```python
from build123d import *

# Parameters (mm, degrees)
SKETCH1_R           = 16.0625
SKETCH1_R_2         = 18.5625
SKETCH1_R_3         = 1.6
SKETCH1_R_4         = 2.35
SKETCH1_R_5         = 2.5625
SKETCH1_R_6         = 7.5625
BOSS_EXTRUDE1_DEPTH = 5
FILLET1_R           = 15
FILLET2_R           = 30


with BuildPart() as part:
    # Sketch1 → Boss-Extrude1 (new body)
    with BuildSketch(Plane.XY):
        Polygon((-20, -31.5), (20, -31.5), (60, -13.814957213), (60, 13.141793742), (20, 31.5), (-20, 8.126584262), align=None)
        Circle(SKETCH1_R, mode=Mode.SUBTRACT)
        with Locations((40, 0)):
            Circle(SKETCH1_R_2, mode=Mode.SUBTRACT)
        with Locations((20, 11.209005776)):
            Circle(SKETCH1_R_3, mode=Mode.SUBTRACT)
        with Locations((20, -9.557095977)):
            Circle(SKETCH1_R_4, mode=Mode.SUBTRACT)
        with Locations((20, 21.918567686)):
            Circle(SKETCH1_R_5, mode=Mode.SUBTRACT)
        with Locations((20, -21.316811866)):
            Circle(SKETCH1_R_6, mode=Mode.SUBTRACT)
        with Locations((0.737105173, -21.316811866)):
            Circle(SKETCH1_R_3, mode=Mode.SUBTRACT)
        with Locations((-4.862894827, -21.316811866)):
            Circle(SKETCH1_R_3, mode=Mode.SUBTRACT)
    extrude(amount=BOSS_EXTRUDE1_DEPTH)

    # Fillet1
    fillet1_edges = [part.edges().sort_by_distance(p)[0] for p in [
        (20, -31.5, 2.5),
        (-20, 8.126584262, 2.5),
        (20, 31.5, 2.5),
        (60, 13.141793742, 2.5),
        (60, -13.814957213, 2.5),
    ]]
    fillet(fillet1_edges, radius=FILLET1_R)

    # Fillet2
    fillet2_edges = [part.edges().sort_by_distance(p)[0] for p in [
        (-20, -31.5, 2.5),
    ]]
    fillet(fillet2_edges, radius=FILLET2_R)


solid = part.part
```
Check sheet for the modelled part. Datum: model origin and axes. Units: mm. Give positions to 0.01 mm unless a question says otherwise; leave off trailing zeros. Order: outer loops, then holes, each group sorted by start corner. A loop starts at its lowest first (then second) coordinate and runs counter-clockwise, first axis right, second up. Notation, with made-up numbers: M 56,44 L 72,44 A22 cw 72,62 Z; hole C 29,-17.75 d3. An arc over 180 degrees is marked long. Answer in a Markdown table with one row per item. Add a question column.
Q1. Sectioned sample at C-C, the plane x = 20. Record the boundary of the cut face in (y, z), and give its area (3 significant figures).
Q2. Sectioned sample at A-A, the plane x = 34.5. Record the boundary of the cut face in (y, z), and give its area (3 significant figures).
Q3. Sectioned sample at B-B, the plane z = 2.9. Count the separate pieces of the cut face and the enclosed holes in it, and give its area (3 significant figures).
Q4. Thickness scan on L1, parallel to Y at x = 20, z = 3; L2, parallel to X at y = 8, z = 2.25; L3, parallel to Y at x = 0, z = 2.4. Record the ranges inside material, lowest first.
Q5. Gauge pin test, flat ends, axial feed: pin 1 Ø19.5 at (x, y) = (0, 0) entering from -Z; pin 2 Ø1 at (y, z) = (-18.5, 2.5) entering from +X; pin 3 Ø1.5 at (x, z) = (-11.5, 4) entering from +Y; pin 4 Ø1.5 at (x, z) = (19.5, 1.5) entering from -Y. Record the tip position at first contact, or that the pin passes through.
Q6. Release check for a two-part mould opening along Y. For faces 1 (the cylindrical face through (-10.979, -22.945, 2.535)), 2 (the cylindrical face through (19.653, 9.647, 2.465)), 3 (the flat face through (0.529, 20.123, 2.465)) record: released by +Y, released by -Y, zero draft, split by the parting line, or undercut.
Q7. Sectioned sample at D-D, the plane x = 0. Record the boundary of the cut face in (y, z), and give its area (3 significant figures).
Verdict:
| question | item | result |
|---|---|---|
| 1 | outline | M -31.16,0 L -28.88,0 L -28.88,5 L -31.16,5 Z; M -13.75,0 L -11.91,0 L -11.91,5 L -13.75,5 Z; M -7.21,0 L 9.61,0 L 9.61,5 L -7.21,5 Z; M 12.81,0 L 19.36,0 L 19.36,5 L 12.81,5 Z; M 24.48,0 L 29.59,0 L 29.59,5 L 24.48,5 Z |
| 1 | area | 163 mm² |
| 2 | outline | M -25.09,0 L -17.73,0 L -17.73,5 L -25.09,5 Z; M 17.73,0 L 24.85,0 L 24.85,5 L 17.73,5 Z |
| 2 | area | 72.4 mm² |
| 3 | separate pieces | 1 |
| 3 | enclosed holes | 8 |
| 3 | area | 1,470 mm² |
| 4 | L1 | -31.16 to -28.88, -13.75 to -11.91, -7.21 to 9.61, 12.81 to 19.36, 24.48 to 29.59 |
| 4 | L2 | -17.37 to -13.93, 13.93 to 23.25, 56.75 to 59.32 |
| 4 | L3 | -29.78 to -22.74, -19.9 to -16.06, 16.06 to 19.81 |
| 5 | pin 1 | through |
| 5 | pin 2 | x = 50.53 |
| 5 | pin 3 | y = 13.53 |
| 5 | pin 4 | y = -31.38 |
| 6 | face 1 | released by -Y |
| 6 | face 2 | undercut |
| 6 | face 3 | released by +Y |
| 7 | outline | M -29.78,0 L -22.74,0 L -22.74,5 L -29.78,5 Z; M -19.9,0 L -16.06,0 L -16.06,5 L -19.9,5 Z; M 16.06,0 L 19.81,0 L 19.81,5 L 16.06,5 Z |
| 7 | area | 73.2 mm² |
